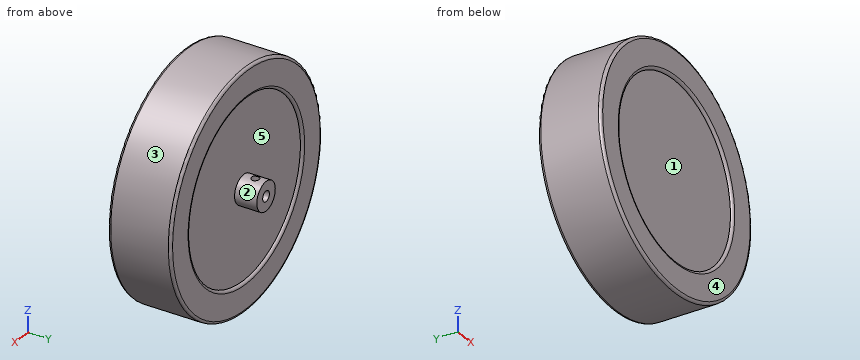
```python
from build123d import *

# Parameters (mm, degrees)
SKETCH2_R           = 90
BOSS_EXTRUDE1_DEPTH = 48
SKETCH3_R           = 67.5
CUT_EXTRUDE1_DEPTH  = 2
CUT_EXTRUDE2_START  = -2
SKETCH4_R           = 67.5
CUT_EXTRUDE2_DEPTH  = 2
FILLET1_R           = 2
SKETCH_1_R          = 11
EXTRUDE_1_DEPTH     = 17
SKETCH_2_R          = 4
CUT_EXTRUDE_1_DEPTH = 15
SKETCH_3_R          = 3
CUT_EXTRUDE_2_DEPTH = 15


with BuildPart() as part:
    # Sketch2 → Boss-Extrude1 (new body)
    with BuildSketch(Plane(origin=(0, 0, 0), x_dir=(1, 0, 0), z_dir=(0, 1, 0))):
        with Locations(Location((0, 0, 0), (0, 0, 270))):
            Circle(SKETCH2_R)
    extrude(amount=BOSS_EXTRUDE1_DEPTH)

    # Sketch3 → Cut-Extrude1 (cut)
    with BuildSketch(Plane(origin=(0, 48, 0), x_dir=(1, 0, 0), z_dir=(0, 1, 0))):
        with Locations(Location((0, 0, 0), (0, 0, 270))):
            Circle(SKETCH3_R)
    extrude(amount=-CUT_EXTRUDE1_DEPTH, mode=Mode.SUBTRACT)

    # Sketch4 → Cut-Extrude2 (cut)
    with BuildSketch(Plane.XZ.offset(CUT_EXTRUDE2_START)):
        with Locations(Location((0, 0, 0), (0, 0, 90))):
            Circle(SKETCH4_R)
    extrude(amount=CUT_EXTRUDE2_DEPTH, mode=Mode.SUBTRACT)

    # Fillet1
    fillet1_edges = [part.edges().sort_by_distance(p)[0] for p in [
        (0, 0, -67.5),
        (0, 0, -90),
        (0, 48, -90),
        (0, 48, -67.5),
    ]]
    fillet(fillet1_edges, radius=FILLET1_R - 0.0001)  # a hair under: the kernel refuses the full size

    # 草图1 → 凸台-拉伸1 (add)
    with BuildSketch(Plane(origin=(0, 46, 0), x_dir=(1, 0, 0), z_dir=(0, 1, 0))):
        with Locations(Location((0, 0, 0), (0, 0, 270))):
            Circle(SKETCH_1_R)
    extrude(amount=EXTRUDE_1_DEPTH)

    # 草图2 → 切除-拉伸1 (cut)
    with BuildSketch(Plane(origin=(0, 63, 0), x_dir=(1, 0, 0), z_dir=(0, 1, 0))):
        with Locations(Location((0, 0, 0), (0, 0, 270))):
            Circle(SKETCH_2_R)
    extrude(amount=-CUT_EXTRUDE_1_DEPTH, mode=Mode.SUBTRACT)

    # 草图3 → 切除-拉伸2 (cut)
    with BuildSketch(Plane.XY):
        with Locations(Location((0, 55, 0), (0, 0, 90.000000006))):
            Circle(SKETCH_3_R)
    extrude(amount=CUT_EXTRUDE_2_DEPTH, mode=Mode.SUBTRACT)


solid = part.part
```
CAD build for the part. Positions are in the model's coordinates, mm. Face numbers are marked on the shaded views. A direction names the side the tool comes from. Coordinates: 2 decimals unless noted, no trailing zeros. Loops run counter-clockwise (first coordinate to the right, second up) from the corner with the lowest first, then second, coordinate; pieces in that order, holes last. Notation, with made-up numbers: (28.25, -37) - (70.25, -37) arc R16 ccw to (70.25, -14) - close; hole circle Ø11 at (23.25, -5.75). An arc over 180 degrees is marked (long way). Use CSV: the item, a comma, the result in double quotes. Start each with the question number.
Q1. Probe probe 1 along Y at (x, z) = (0, 6); probe 2 along X at (y, z) = (55, 0); probe 3 along Y at (x, z) = (16, 5). List the from-to ranges inside material, lowest first. Write a range as from..to.
Q2. Cut at D-D, the plane y = 55. List the corners of the cut face in (x, z).
Q3. Two-plate mould, pull along Z, no slides. Class the marked faces 3, 4 and 5: +Z half, -Z half, draft (parallel to the pull), parting line (faces both ways), or undercut.
Q4. 3-axis set-ups, long thin cutter, end or side, ignore diameter. For the marked faces 1 and 2: which of +Z, -Z, +X, -X, +Y, -Y reach the whole face in a straight line?
Q5. Drop flat-ended pins along their axis: P1, Ø2, axis at x = 28.5, y = 21, coming from the -Z side; P2, Ø1.5, axis at x = 51.5, y = 24.5, coming from the +Z side; P3, Ø5, axis at x = 0, y = 55, coming from the +Z side; P4, Ø3, axis at x = -68, z = -29.5, coming from the -Y side. Give the stop position or say it passes through.
Q6. Cut at C-C, the plane y = 19. List the corners of the cut face in (x, z).
Here are the results:
1,probe 1,"2..52, 58..63"
1,probe 2,"-11..-4, 4..11"
1,probe 3,"2..46"
2,outline,"(-3, 2.65) - (-3, 10.58) arc R11 ccw (long way) to (3, 10.58) - (3, 2.65) arc R4 cw (long way) to start"
3,face 3,"parting line"
3,face 4,"draft"
3,face 5,"undercut"
4,face 1,"-Y"
4,face 2,"+Y"
5,P1,"z = -85.7"
5,P2,"z = 74.33"
5,P3,"z = -3.12"
5,P4,"y = 0"
6,outline,"circle Ø180 at (0, 0)"
